Model file for the job. Use its own axes, mm. A direction names the side the tool comes from. Round coordinates to 2 decimals unless told otherwise and drop trailing zeros. Loops run counter-clockwise (first coordinate to the right, second up) from the corner with the lowest first, then second, coordinate; pieces in that order, holes last. Notation, with made-up numbers: (-13.5, 19.25) -> (-0.5, 19.25) arc R30 cw to (-0.5, 48.25) -> close; hole circle Ø11 at (72.5, 18). An arc over 180 degrees is marked (long way). Use a Markdown table: item, result. Add a question column.
```python
from build123d import *

# Parameters (mm, degrees)
ESBO_O1_W                = 65
ESBO_O1_H                = 50
RESSALTO_EXTRUS_O1_DEPTH = 2
ESBO_O2_W                = 50
ESBO_O2_H                = 50
RESSALTO_EXTRUS_O2_DEPTH = 2
ESBO_O3_W                = 50
ESBO_O3_H                = 2
RESSALTO_EXTRUS_O3_DEPTH = 10
ESBO_O4_R                = 1.5
CORTE_EXTRUS_O1_DEPTH    = 51
ESBO_O5_R                = 16
ESBO_O5_R_2              = 2.5
CORTE_EXTRUS_O2_DEPTH    = 10
ESBO_O6_R                = 2
CORTE_EXTRUS_O3_DEPTH    = 10


with BuildPart() as part:
    # Esboço1 → Ressalto-extrusão1 (new body)
    with BuildSketch(Plane(origin=(0, 0, 0), x_dir=(1, 0, 0), z_dir=(0, 1, 0))):
        Rectangle(ESBO_O1_W, ESBO_O1_H)
    extrude(amount=-RESSALTO_EXTRUS_O1_DEPTH)

    # Esboço2 → Ressalto-extrusão2 (add)
    with BuildSketch(Plane.ZY.offset(32.5)):
        with Locations((0, -25)):
            Rectangle(ESBO_O2_W, ESBO_O2_H)
    ressalto_extrus_o2 = extrude(amount=-RESSALTO_EXTRUS_O2_DEPTH)

    # Esboço3 → Ressalto-extrusão3 (add)
    with BuildSketch(Plane(origin=(-30.5, 0, 0), x_dir=(0, 0, -1), z_dir=(1, 0, 0))):
        with Locations((0, -49)):
            Rectangle(ESBO_O3_W, ESBO_O3_H)
    ressalto_extrus_o3 = extrude(amount=RESSALTO_EXTRUS_O3_DEPTH)

    # Espelhar1: Ressalto-extrusão2, Ressalto-extrusão3 across plane
    add(ressalto_extrus_o2.mirror(Plane(origin=(0, 0, 0), x_dir=(0, 0, 1), z_dir=(1, 0, 0))))
    add(ressalto_extrus_o3.mirror(Plane(origin=(0, 0, 0), x_dir=(0, 0, 1), z_dir=(1, 0, 0))))

    # Esboço4 → Corte-extrusão1 (cut, through all)
    with BuildSketch(Plane(origin=(0, 0, 0), x_dir=(1, 0, 0), z_dir=(0, 1, 0))):
        with Locations((-15.5, 15.5)):
            Circle(ESBO_O4_R)
        with Locations((-15.5, -15.5)):
            Circle(ESBO_O4_R)
        with Locations((15.5, -15.5)):
            Circle(ESBO_O4_R)
        with Locations((15.5, 15.5)):
            Circle(ESBO_O4_R)
    extrude(amount=-CORTE_EXTRUS_O1_DEPTH, mode=Mode.SUBTRACT)

    # Esboço5 → Corte-extrusão2 (cut)
    with BuildSketch(Plane(origin=(0, 0, 0), x_dir=(1, 0, 0), z_dir=(0, 1, 0))):
        Circle(ESBO_O5_R)
        Circle(ESBO_O5_R_2, mode=Mode.SUBTRACT)
        Circle(ESBO_O5_R_2)
    extrude(amount=-CORTE_EXTRUS_O2_DEPTH, mode=Mode.SUBTRACT)

    # Esboço6 → Corte-extrusão3 (cut)
    with BuildSketch(Plane(origin=(0, -48, 0), x_dir=(1, 0, 0), z_dir=(0, 1, 0))):
        with Locations((-25.5, -15)):
            Circle(ESBO_O6_R)
        with Locations((25.5, -15)):
            Circle(ESBO_O6_R)
        with Locations((25.5, 15)):
            Circle(ESBO_O6_R)
        with Locations((-25.5, 15)):
            Circle(ESBO_O6_R)
    extrude(amount=-CORTE_EXTRUS_O3_DEPTH, mode=Mode.SUBTRACT)


solid = part.part
```
1) Cut at A-A on y = -12. Write the cut outline in (x, z), and give its area (3 significant figures).
2) Cut at D-D on x = 15. Write the cut outline in (y, z).
3) Pin check, flat tips, straight feed: pin 1 Ø2.5 at (x, z) = (15.5, -15.5) entering from -Y; pin 2 Ø3.5 at (x, z) = (-15.5, 15.5) entering from -Y. Stop position of each tip, or through.
4) Wall check: probe 1 along Z at (x, y) = (25.5, -49.6); probe 2 along Y at (x, z) = (23.5, 11.5); probe 3 along X at (y, z) = (-3, -11). Give the ranges that are in metal, low to high. Write a range as from..to.
5) Tool access for faces 4 (the face through (-30.5, -25, 0)), 5 (the face through (0, -1, 25)), 6 (the face through (24.026, -48.986, 13.648)), 7 (the face through (20.5, -49, 0)), 8 (the face through (-15, 0, -6)): list every direction of +Z, -Z, +X, -X, +Y, -Y with a clear straight run to the whole face (end or side of a thin tool).
6) Pull direction Z, two halves, no side cores. Call faces 1 (the face through (0, -1, -25)), 2 (the face through (-17, -0.99, 15.43)), 3 (the face through (-27, -50, 0)): +Z half, -Z half, draft (parallel to the pull), parting line (faces both ways), or undercut.
7) Cut at B-B on z = 0. Write the cut outline in (x, y), and give its area (3 significant figures).
8) Cut at C-C on x = 0. Write the cut outline in (y, z).
Established:
| question | item | result |
|---|---|---|
| 1 | outline | (-32.5, -25) -> (-30.5, -25) -> (-30.5, 25) -> (-32.5, 25) -> close; (30.5, -25) -> (32.5, -25) -> (32.5, 25) -> (30.5, 25) -> close |
| 1 | area | 200 mm^2 |
| 2 | outline | (-2, -25) -> (0, -25) -> (0, -16.91) -> (-2, -16.91) -> close; (-2, -14.09) -> (0, -14.09) -> (0, -5.57) -> (-2, -5.57) -> close; (-2, 5.57) -> (0, 5.57) -> (0, 14.09) -> (-2, 14.09) -> close; (-2, 16.91) -> (0, 16.91) -> (0, 25) -> (-2, 25) -> close |
| 3 | pin 1 | passes through |
| 3 | pin 2 | stops at y = -2 |
| 4 | probe 1 | z = -25..-17, -13..13, 17..25 |
| 4 | probe 2 | y = -50..-48, -2..0 |
| 4 | probe 3 | x = -32.5..-30.5, 30.5..32.5 |
| 5 | face 4 | +Z, -Z |
| 5 | face 5 | +Z, +X, -X, +Y, -Y |
| 5 | face 6 | -Y |
| 5 | face 7 | +Z, -Z, -Y |
| 5 | face 8 | +Z, -Z, +X, -X, +Y |
| 6 | face 1 | -Z half |
| 6 | face 2 | undercut |
| 6 | face 3 | draft |
| 7 | outline | (-32.5, -50) -> (-20.5, -50) -> (-20.5, -48) -> (-30.5, -48) -> (-30.5, -2) -> (-16, -2) -> (-16, 0) -> (-32.5, 0) -> close; (16, -2) -> (30.5, -2) -> (30.5, -48) -> (20.5, -48) -> (20.5, -50) -> (32.5, -50) -> (32.5, 0) -> (16, 0) -> close |
| 7 | area | 298 mm^2 |
| 8 | outline | (-2, -25) -> (0, -25) -> (0, -16) -> (-2, -16) -> close; (-2, 16) -> (0, 16) -> (0, 25) -> (-2, 25) -> close |
